Here's the drawing with two shaded views (mm, measured from the low corner). I have some questions. Give positions to 0.01 mm unless a question says otherwise; leave off trailing zeros. Write each loop counter-clockwise with the first axis right and the second up, starting at its lowest first coordinate (ties: lowest second). Pieces come first, ordered by that corner, then holes. Notation, with made-up numbers: M -5.75,82.25 L 39.25,82.25 A29 cw 39.25,120.25 Z; hole C 33.25,53 d7. An arc over 180 degrees is marked long. Use one line per item in the form item = value.
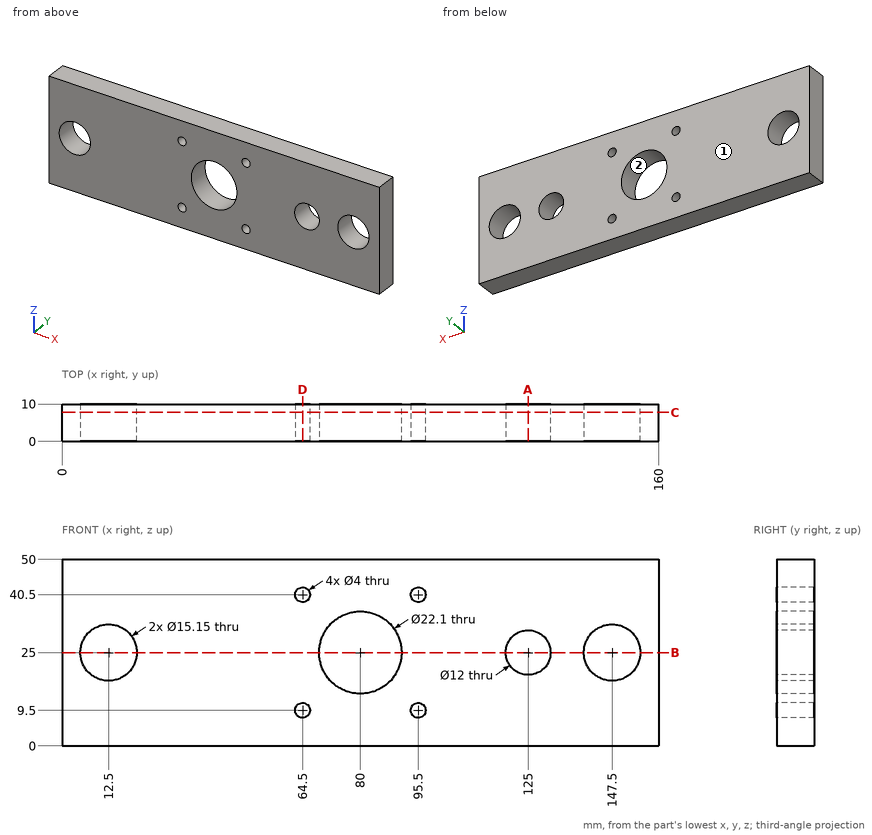
1) I want a section at A-A, the plane x = 125. Please give me the cut outline in (y, z), plus the area to 3 significant figures.
Checked values:
outline = M 0,0 L 10,0 L 10,19 L 0,19 Z; M 0,31 L 10,31 L 10,50 L 0,50 Z
area = 380 mm2
2) I want a section at C-C, the plane y = 7.75. Count the separate pieces of the cut face and the enclosed holes in it, plus the area to 3 significant figures.
Checked values:
separate_pieces = 1
enclosed_holes = 8
area = 7,090 mm2
3) For pin 1 Ø12 at (x, z) = (147.5, 25) entering from +Y, with a flat end and sliding along its axis, tell me the tip position at first contact or that it passes through.
Checked values:
pin_1 = through
4) I want a section at B-B, the plane z = 25. Please give me the cut outline in (x, y) (3 decimals), plus the area to 3 significant figures.
Checked values:
outline = M 0,0 L 4.925,0 L 4.925,10 L 0,10 Z; M 20.075,0 L 68.95,0 L 68.95,10 L 20.075,10 Z; M 91.05,0 L 119,0 L 119,10 L 91.05,10 Z; M 131,0 L 139.925,0 L 139.925,10 L 131,10 Z; M 155.075,0 L 160,0 L 160,10 L 155.075,10 Z
area = 956 mm2
5) I want a section at D-D, the plane x = 64.5. Please give me the cut outline in (y, z), plus the area to 3 significant figures.
Checked values:
outline = M 0,0 L 10,0 L 10,7.5 L 0,7.5 Z; M 0,11.5 L 10,11.5 L 10,38.5 L 0,38.5 Z; M 0,42.5 L 10,42.5 L 10,50 L 0,50 Z
area = 420 mm2
6) Thinking about a two-plate mould opening in Z: for the marked faces 1 and 2, which applies, released by +Z, released by -Z, zero draft, split by the parting line, or undercut?
Checked values:
face_1 = zero draft
face_2 = undercut
7) If I drill on L1, parallel to X at y = 7, z = 40.5; L2, parallel to Z at x = 95.5, y = 6.25; L3, parallel to Z at x = 125, y = 6.5, over which ranges is the centre line in solid material (lowest first)?
Checked values:
L1 = 0 to 62.5, 66.5 to 93.5, 97.5 to 160
L2 = 0 to 7.5, 11.5 to 38.5, 42.5 to 50
L3 = 0 to 19, 31 to 50
